Read the model definition and answer for the solid it produces. Units are mm, in the model's axes. Face numbers are marked on the shaded views. A direction names the side the tool comes from. Coordinates: 2 decimals unless noted, no trailing zeros. Loops run counter-clockwise (first coordinate to the right, second up) from the corner with the lowest first, then second, coordinate; pieces in that order, holes last. Notation, with made-up numbers: (-33, 24.5) - (5, 24.5) arc R31 ccw to (5, 53.5) - close; hole circle Ø2 at (68.25, 3). An arc over 180 degrees is marked (long way). Use one line per item in the form item = value. Start each with the question number.
1) A cutting plane is placed at A-A (y = 1.75). Give the vertices of the cut face in (x, z), and give its area (3 significant figures).
2) A cutting plane is placed at C-C (z = 22). Give the vertices of the cut face in (x, y).
3) Consider line 1 (X direction, y = -4, z = 10.5); line 2 (Z direction, x = 15, y = -9.5); line 3 (Z direction, x = 33.5, y = -10.5). Determine where each line is inside the solid, lowest interval first.
4) A cutting plane is placed at D-D (z = 4). Give the vertices of the cut face in (x, y).
5) Which of the six approach directions +Z, -Z, +X, -X, +Y, -Y give full straight-line access (tool end or side, diameter ignored) to the marked faces 1, 2 and 3?
6) A cutting plane is placed at B-B (x = -23). Give the vertices of the cut face in (y, z), and give its area (3 significant figures).
7) The mould has two halves that part along Z. Classify the marked faces 4, 5, 6 and 7: released by +Z, released by -Z, zero draft, split by the parting line, or undercut.
8) Each of these flat-tipped pins is pushed along its axis until it touches: P1, Ø3, axis at x = 1, y = -8.5, coming from the +Z side; P2, Ø4, axis at x = -9, y = -8, coming from the +Z side; P3, Ø8, axis at x = -32, y = 10, coming from the +Z side. Where does it stop, or does it pass through?
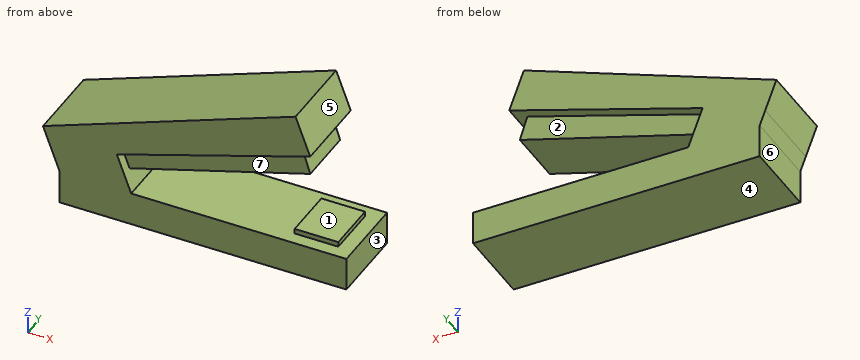
from build123d import *

# Parameters (mm, degrees)
F2_DEPTH = 12.7
F3_DEPTH = 9.3243
F4_W     = 14.10933
F4_H     = 16.725193
F5_DEPTH = 1.62709


with BuildPart() as f2:
    # F0 (on Front) → F2 (new body, symmetric)
    with BuildSketch(Plane.XZ):
        Polygon((-50.360113, 15.644414), (-48.572179, 10.876591), (-25.479328, 10.876591), (-30.114328, 23.236587), align=None)
        Polygon((-25.479328, 10.876591), (-48.572179, 10.876591), (-48.572179, 0), (44.102348, 0), (44.102348, 10.876591), align=None)
        Polygon((-53.984965, 25.31068), (-50.360113, 15.644414), (-30.114328, 23.236587), (32.39506, 43.287981), (27.655806, 55.925984), align=None)
    extrude(amount=F2_DEPTH, both=True)

    # F1 (on Front) → F3 (join, symmetric)
    with BuildSketch(Plane.XZ):
        Polygon((30.692847, 34.417707), (28.308937, 41.867431), (-30.041804, 23.617359), (-28.010949, 16.836369), align=None)
    extrude(amount=F3_DEPTH, both=True)

    # F4 (on face) → F5 (join)
    with BuildSketch(Plane.XY.offset(10.876591)):
        with Locations((32.239902, -0.102639)):
            Rectangle(F4_W, F4_H)
    extrude(amount=F5_DEPTH)


solid = f2.part
Found:
q1.outline = (-53.98, 25.31) - (-50.36, 15.64) - (-48.57, 10.88) - (-48.57, 0) - (44.1, 0) - (44.1, 10.88) - (39.29, 10.88) - (39.29, 12.5) - (25.19, 12.5) - (25.19, 10.88) - (-25.48, 10.88) - (-27.74, 16.92) - (30.69, 34.42) - (28.31, 41.87) - (14.6, 37.58) - (32.4, 43.29) - (27.66, 55.93) - close; hole (-30.11, 23.24) - (-29.19, 20.77) - (-29.94, 23.29) - close
q1.area = 2,680 mm^2
q2.outline = (-52.74, -12.7) - (-29.65, -12.7) - (-29.65, 12.7) - (-52.74, 12.7) - close; (-29.56, -9.32) - (-10.77, -9.32) - (-10.77, 9.32) - (-29.56, 9.32) - close
q3.line_1 = -48.57 to 44.1
q3.line_2 = 0 to 10.88, 37.71 to 51.18
q3.line_3 = 0 to 10.88
q4.outline = (-48.57, -12.7) - (44.1, -12.7) - (44.1, 12.7) - (-48.57, 12.7) - close
q5.face_1 = +X, +Y, -Y
q5.face_2 = +X, +Y
q5.face_3 = +Z, -Z, +X, +Y, -Y
q6.outline = (-12.7, 0) - (12.7, 0) - (12.7, 10.88) - (-12.7, 10.88) - close; (-12.7, 25.52) - (-9.32, 25.52) - (-9.32, 18.34) - (9.32, 18.34) - (9.32, 25.52) - (12.7, 25.52) - (12.7, 36.93) - (-12.7, 36.93) - close
q6.area = 700 mm^2
q7.face_4 = released by -Z
q7.face_5 = released by +Z
q7.face_6 = zero draft
q7.face_7 = undercut
q8.P1 = 46.49
q8.P2 = 42.93
q8.P3 = 35.06
